Check sheet for the drawn part. Datum: minimum x, y, z corner. Units: mm. A direction names the side the tool comes from. Coordinates: 2 decimals unless noted, no trailing zeros. Loops run counter-clockwise (first coordinate to the right, second up) from the corner with the lowest first, then second, coordinate; pieces in that order, holes last.
Q1. Access from +Z, -Z, +X, -X, +Y, -Y to the whole of each face (thin tool, end or side, straight path). Record for the marked faces 1, 2 and 3.
Q2. Sectioned sample at B-B (x = 7.5). Enter the section's corners in (y, z), then the cut area to 3 significant figures.
Q3. Sectioned sample at C-C (z = 9). Enter the section's corners in (x, y), then the cut area to 3 significant figures.
Q4. Go/stop test with flat-tipped pins: P1, Ø2, axis at x = 13.5, y = 10.5, coming from the +Z side; P2, Ø1.6, axis at x = 4.5, z = 1, coming from the +Y side; P3, Ø6, axis at x = 8.5, y = 9.5, coming from the +Z side; P4, Ø4, axis at x = 7.5, y = 10, coming from the +Z side. Record where each tip stops, or that it passes through.
Q5. Sectioned sample at D-D (y = 2.5). Enter the section's corners in (x, z), then the cut area to 4 significant figures.
Q6. Sectioned sample at A-A (y = 10). Enter the section's corners in (x, z), then the cut area to 3 significant figures.
Q7. Material ranges on probe 1 along Y at (x, z) = (8.5, 11.75); probe 2 along X at (y, z) = (10, 8.75); probe 3 along Y at (x, z) = (3.25, 14.25), recorded low to high.
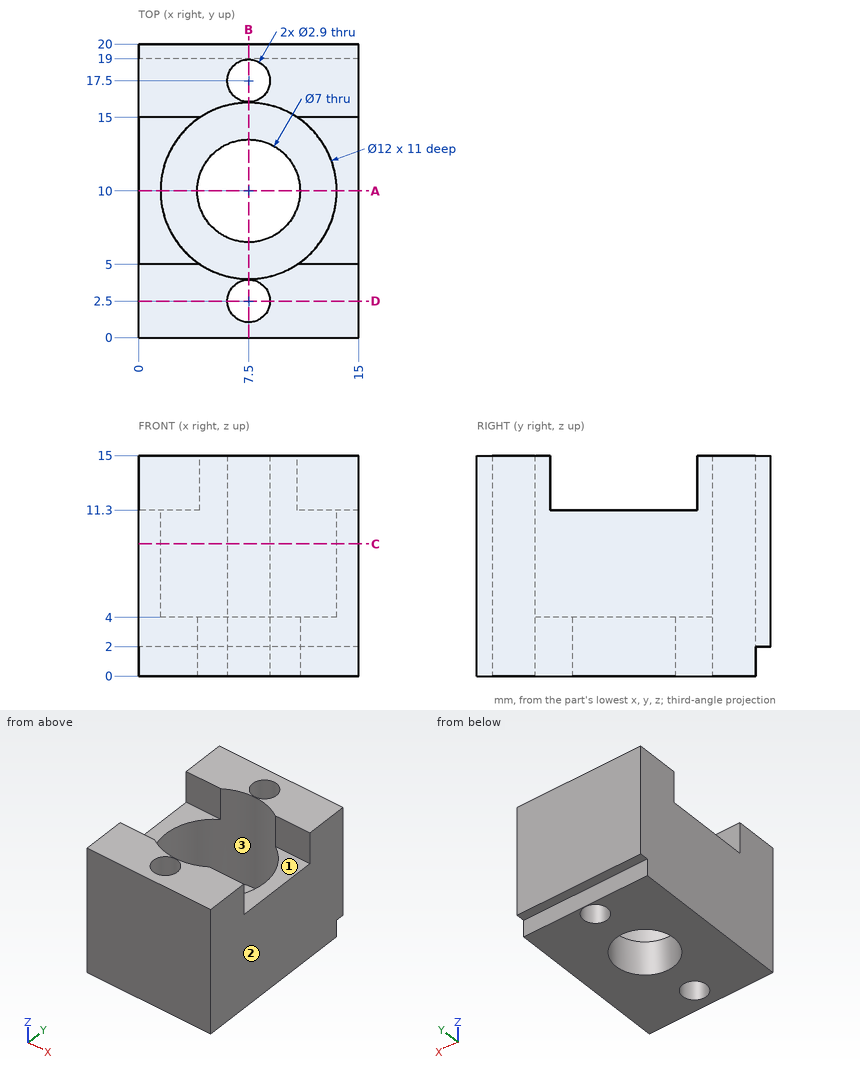
Geometry check:
1. face 1: +Z, +X, -X
1. face 2: +Z, -Z, +X, +Y, -Y
1. face 3: +Z
2. outline: (0, 0) - (1.05, 0) - (1.05, 15) - (0, 15) - close; (3.95, 0) - (6.5, 0) - (6.5, 4) - (4, 4) - (4, 15) - (3.95, 15) - close; (13.5, 0) - (16.05, 0) - (16.05, 15) - (16, 15) - (16, 4) - (13.5, 4) - close; (18.95, 0) - (19, 0) - (19, 2) - (20, 2) - (20, 15) - (18.95, 15) - close
2. area: 51.0 mm2
3. outline: (0, 0) - (15, 0) - (15, 20) - (0, 20) - close; hole circle Ø12 at (7.5, 10); hole circle Ø2.9 at (7.5, 2.5); hole circle Ø2.9 at (7.5, 17.5)
3. area: 174 mm2
4. P1: stops at z = 11.3
4. P2: stops at y = 19
4. P3: stops at z = 4
4. P4: passes through
5. outline: (0, 0) - (6.05, 0) - (6.05, 15) - (0, 15) - close; (8.95, 0) - (15, 0) - (15, 15) - (8.95, 15) - close
5. area: 181.5 mm2
6. outline: (0, 0) - (4, 0) - (4, 4) - (1.5, 4) - (1.5, 11.3) - (0, 11.3) - close; (11, 0) - (15, 0) - (15, 11.3) - (13.5, 11.3) - (13.5, 4) - (11, 4) - close
6. area: 53.9 mm2
7. probe 1: y = 0 to 1.45, 3.55 to 4.08, 15.92 to 16.45, 18.55 to 20
7. probe 2: x = 0 to 1.5, 13.5 to 15
7. probe 3: y = 0 to 5, 15 to 20
